Read the model definition and answer for the solid it produces. Units are mm, in the model's axes. A direction names the side the tool comes from. Coordinates: 2 decimals unless noted, no trailing zeros. Write each loop counter-clockwise with the first axis right and the second up, starting at its lowest first coordinate (ties: lowest second). Pieces come first, ordered by that corner, then holes. Notation, with made-up numbers: (64, 27.25) - (94, 27.25) arc R22 ccw to (94, 34.25) - close; hole circle Ø7 at (65, -7.75). An arc over 180 degrees is marked (long way). Return JSON: item names as keys, results as strings.
```python
from build123d import *

# Parameters (mm, degrees)
SKETCH_1_R       = 5
EXTRUDE_1_DEPTH  = 37
SKETCH_2_R       = 2.5
EXTRUDE_2_DEPTH  = 8
EXTRUDE_3_DEPTH  = 8
CHAMFER_1_SIZE   = 2.5
CHAMFER_1_SIZE_2 = 4.330127019


with BuildPart() as part:
    # 草图1 → 凸台-拉伸1 (new body)
    with BuildSketch(Plane(origin=(0, 0, 0), x_dir=(0, 0, -1), z_dir=(1, 0, 0))):
        Circle(SKETCH_1_R)
    extrude(amount=EXTRUDE_1_DEPTH)

    # 草图2 → 凸台-拉伸2 (add)
    with BuildSketch(Plane(origin=(37, 0, 0), x_dir=(0, 0, -1), z_dir=(1, 0, 0))):
        Circle(SKETCH_2_R)
    extrude(amount=EXTRUDE_2_DEPTH)

    # 草图3 → 凸台-拉伸3 (add)
    with BuildSketch(Plane.ZY):
        Polygon((0, 3.535533906), (-3.535533906, 0), (0, -3.535533906), (3.535533906, 0), align=None)
    extrude(amount=EXTRUDE_3_DEPTH)

    # 倒角1
    # the kernel refuses this chamfer: 4.330127019, 2.5 mm, written as the material it takes off along each edge
    with BuildSketch(Plane(origin=(37, 0, 0), x_dir=(0, 0, -1), z_dir=(0, -1, 0))) as chamfer_1_piece_1_section:
        Polygon((5, -CHAMFER_1_SIZE), (5 - CHAMFER_1_SIZE_2, 0), (5, 0), align=None)
    chamfer_1_piece_1 = revolve(axis=Axis((37, 0, 0), (1, 0, 0)), mode=Mode.PRIVATE)
    chamfer_1_piece_1 = chamfer_1_piece_1 - Plane(origin=(35.221489766, 0, 0), x_dir=(0, 0, -1), z_dir=(-1, 0, 0)) * Cylinder(2.5, 20, mode=Mode.PRIVATE)
    add(chamfer_1_piece_1, mode=Mode.SUBTRACT)


solid = part.part
```
(1) Straight lines are drawn through the part: line 1 (Z direction, x = 31, y = 0.25); line 2 (Y direction, x = 25, z = -2); line 3 (Z direction, x = 16, y = 1). For each, find the intervals that lie inside material, in ascending order. Write a range as from..to.
Answer:
{"line 1": "-4.99..4.99", "line 2": "-4.58..4.58", "line 3": "-4.9..4.9"}
(2) Flat-ended cylindrical pins translate along their axes: P1, Ø2, axis at x = 3.5, z = 4, coming from the +Y side; P2, Ø2, axis at x = 3.5, y = 1.5, coming from the -Z side; P3, Ø4, axis at x = 25.5, z = 2.5, coming from the +Y side. Find the tip coordinate at first contact, or state that the pin passes through.
Answer:
{"P1": "y = 4", "P2": "z = -4.97", "P3": "y = 4.97"}
(3) Which of the six approach directions +Z, -Z, +X, -X, +Y, -Y give full straight-line access (tool end or side, diameter ignored) to faces 1 (the face through (40.41, 2.44, 0.54)), 2 (the face through (-3.944, 1.743, 1.793)), 3 (the face through (0, -2, -2)), 4 (the face through (-3.944, 1.793, -1.743))?
Answer:
{"face 1": "+X", "face 2": "+Z, -X, +Y", "face 3": "-X", "face 4": "-Z, -X, +Y"}
(4) A cutting plane is placed at A-A (x = 6.5). Determine the outline of the cut face in (y, z), and give its area (3 significant figures).
Answer:
{"outline": "circle Ø10 at (0, 0)", "area": "78.5 mm²"}
